Part model, mm, in its own coordinate system. A direction names the side the tool comes from. Give positions to 0.01 mm unless a question says otherwise; leave off trailing zeros. Order: outer loops, then holes, each group sorted by start corner. A loop starts at its lowest first (then second) coordinate and runs counter-clockwise, first axis right, second up. Notation, with made-up numbers: M 34,-28.5 L 84,-28.5 A21 cw 84,-14.5 Z; hole C 49,20.5 d1. An arc over 180 degrees is marked long. Answer as a JSON object with one key per item and string values.
from build123d import *

# Parameters (mm, degrees)
BOSS_EXTRUDE1_DEPTH     = 10.8
CUT_EXTRUDE1_DEPTH      = 63.509359299
CUT_EXTRUDE1_DEPTH_BACK = 63.509359299
SKETCH14_W              = 32
SKETCH14_H              = 30
CUT_EXTRUDE3_DEPTH      = 60.51688836
FILLET1_R               = 3
SKETCH16_R              = 1.6
CUT_EXTRUDE2_DEPTH      = 60.51688836
CUT_EXTRUDE4_DEPTH      = 75.590213715
BOSS_EXTRUDE3_START     = -2.5
BOSS_EXTRUDE3_OUTLINE_R = 1.65
BOSS_EXTRUDE3_DEPTH     = 2.5
BOSS_EXTRUDE4_START     = 7.1
SKETCH24_R              = 3.6
SKETCH24_R_2            = 1.6
BOSS_EXTRUDE4_DEPTH     = 7.1
CHAMFER1_SIZE           = 1


# Read off the part's stored shape, not the designer's step: Boss-Extrude3
with BuildPart() as part:
    # Sketch6 → Revolve1 (revolve)
    with BuildSketch(Plane(origin=(0, 0, 0), x_dir=(0, 0, -1), z_dir=(1, 0, 0)), mode=Mode.PRIVATE) as revolve1_sk:
        Polygon((-2, 25.4), (-2, 35.1), (-25, 35.1), (-25, 37.95), (-12, 37.95), (-12, 41.1), (-9.5, 41.1), (-9.5, 38.1), (0, 38.1), (0, 25.4), (0, 0), (-2, 0), align=None)
    revolve(revolve1_sk.sketch.rotate(Axis((0, 0, 0), (0, 0, 1)), 90), axis=Axis((0, 0, 0), (0, 0, 1)))

    # Sketch15 → Boss-Extrude1 (add)
    with BuildSketch(Plane.XY.offset(2)):
        with BuildLine():
            Line((-20, 15.904297927), (20, 15.904297927))
            ThreePointArc((20, 15.904297927), (22.121320344, 15.02561827), (23, 12.904297927))
            Line((23, 12.904297927), (23, -24.995702073))
            ThreePointArc((23, -24.995702073), (22.121320344, -27.117022417), (20, -27.995702073))
            Line((20, -27.995702073), (-20, -27.995702073))
            ThreePointArc((-20, -27.995702073), (-22.121320344, -27.117022417), (-23, -24.995702073))
            Line((-23, -24.995702073), (-23, 12.904297927))
            ThreePointArc((-23, 12.904297927), (-22.121320344, 15.02561827), (-20, 15.904297927))
        make_face()
    extrude(amount=BOSS_EXTRUDE1_DEPTH)

    # Sketch14 → Cut-Extrude1 (cut, two sides: drawn at the far end of the back side and taken through both)
    with BuildSketch(Plane.XY.offset(2).offset(-CUT_EXTRUDE1_DEPTH_BACK)):
        with Locations((-0.00164643, -5.995702073)):
            Rectangle(SKETCH14_W, SKETCH14_H)
    extrude(amount=CUT_EXTRUDE1_DEPTH + CUT_EXTRUDE1_DEPTH_BACK, mode=Mode.SUBTRACT)

    # Sketch18 → Cut-Extrude3 (cut, through all)
    with BuildSketch(Plane.XY.offset(12.8)):
        with BuildLine():
            Line((19.99835357, -24.995702073), (23.99835357, -24.995702073))
            Line((23.99835357, -24.995702073), (23.99835357, -25.995702073))
            ThreePointArc((23.99835357, -25.995702073), (23.119673914, -28.117022417), (20.99835357, -28.995702073))
            Line((20.99835357, -28.995702073), (19.99835357, -28.995702073))
            Line((19.99835357, -28.995702073), (19.99835357, -24.995702073))
        make_face()
        with BuildLine():
            Line((-20.00164643, -24.995702073), (-24.00164643, -24.995702073))
            Line((-24.00164643, -24.995702073), (-24.00164643, -25.995702073))
            ThreePointArc((-24.00164643, -25.995702073), (-23.122966774, -28.117022417), (-21.00164643, -28.995702073))
            Line((-21.00164643, -28.995702073), (-20.00164643, -28.995702073))
            Line((-20.00164643, -28.995702073), (-20.00164643, -24.995702073))
        make_face()
    extrude(amount=CUT_EXTRUDE3_DEPTH, mode=Mode.SUBTRACT)

    # Fillet1
    fillet1_edges = [part.edges().sort_by_distance(p)[0] for p in [
        (-16.00164643, 9.004297927, 6.4),
        (-16.00164643, -20.995702073, 6.4),
        (15.99835357, -20.995702073, 6.4),
        (15.99835357, 9.004297927, 6.4),
    ]]
    fillet(fillet1_edges, radius=FILLET1_R)

    # Sketch16 → Cut-Extrude2 (cut, through all)
    with BuildSketch(Plane.XY.offset(12.8)):
        with Locations((-20.00164643, 13.004297927)):
            Circle(SKETCH16_R)
        with Locations((-20.00164643, -24.995702073)):
            Circle(SKETCH16_R)
        with Locations((19.99835357, -24.995702073)):
            Circle(SKETCH16_R)
        with Locations((19.99835357, 13.004297927)):
            Circle(SKETCH16_R)
    extrude(amount=-CUT_EXTRUDE2_DEPTH, mode=Mode.SUBTRACT)

    # Sketch20 → Cut-Extrude4 (cut, through all)
    with BuildSketch(Plane(origin=(0, 15.904297927, 0), x_dir=(1, 0, 0), z_dir=(0, 1, 0))):
        Polygon((20, -12.8), (-20, -12.8), (-20, -25), (19.99835357, -25), align=None)
    extrude(amount=CUT_EXTRUDE4_DEPTH, mode=Mode.SUBTRACT)

    # Boss-Extrude3 outline → Boss-Extrude3 (add)
    # profile 1 of 2: a face of its own
    with BuildSketch(Plane.XY.offset(12).offset(BOSS_EXTRUDE3_START)):
        with BuildLine():
            Line((-26.863244514, 31.105885201), (-34.641419107, 38.884059794))
            Line((-34.641419107, 38.884059794), (-38.884059794, 34.641419107))
            Line((-38.884059794, 34.641419107), (-31.105885201, 26.863244514))
            ThreePointArc((-31.105885201, 26.863244514), (-29.062088707, 29.062088707), (-26.863244514, 31.105885201))
        make_face()
        with Locations((-34.641419107, 34.641419107)):
            Circle(BOSS_EXTRUDE3_OUTLINE_R, mode=Mode.SUBTRACT)
    # profile 2 of 2: a face of its own
    with BuildSketch(Plane.XY.offset(12).offset(BOSS_EXTRUDE3_START)):
        with BuildLine():
            Line((34.641419107, 38.884059794), (26.863244514, 31.105885201))
            ThreePointArc((26.863244514, 31.105885201), (29.062088707, 29.062088707), (31.105885201, 26.863244514))
            Line((31.105885201, 26.863244514), (38.884059794, 34.641419107))
            Line((38.884059794, 34.641419107), (34.641419107, 38.884059794))
        make_face()
        with Locations((34.641419107, 34.641419107)):
            Circle(BOSS_EXTRUDE3_OUTLINE_R, mode=Mode.SUBTRACT)
    boss_extrude3 = extrude(amount=BOSS_EXTRUDE3_DEPTH)

    # Sketch24 → Boss-Extrude4 (add)
    # profile 1 of 4: a face of its own
    with BuildSketch(Plane.XY.offset(12.8).offset(BOSS_EXTRUDE4_START)):
        with Locations(Location((-20.00164643, 13.004297927, 0), (0, 0, 213.6046846))):
            Circle(SKETCH24_R)
        with Locations((-20.00164643, 13.004297927)):
            Circle(SKETCH24_R_2, mode=Mode.SUBTRACT)
    # profile 2 of 4: a face of its own
    with BuildSketch(Plane.XY.offset(12.8).offset(BOSS_EXTRUDE4_START)):
        with Locations(Location((19.99835357, 13.004297927, 0), (0, 0, 126.336057515))):
            Circle(SKETCH24_R)
        with Locations((19.99835357, 13.004297927)):
            Circle(SKETCH24_R_2, mode=Mode.SUBTRACT)
    # profile 3 of 4: a face of its own
    with BuildSketch(Plane.XY.offset(12.8).offset(BOSS_EXTRUDE4_START)):
        with Locations(Location((-20.00164643, -24.995702073, 0), (0, 0, 198.741091164))):
            Circle(SKETCH24_R)
        with Locations((-20.00164643, -24.995702073)):
            Circle(SKETCH24_R_2, mode=Mode.SUBTRACT)
    # profile 4 of 4: a face of its own
    with BuildSketch(Plane.XY.offset(12.8).offset(BOSS_EXTRUDE4_START)):
        with Locations(Location((19.99835357, -24.995702073, 0), (0, 0, 236.442690237))):
            Circle(SKETCH24_R)
        with Locations((19.99835357, -24.995702073)):
            Circle(SKETCH24_R_2, mode=Mode.SUBTRACT)
    extrude(amount=-BOSS_EXTRUDE4_DEPTH)

    # Chamfer1
    chamfer1_edges = [part.edges().sort_by_distance(p)[0] for p in [
        (-21.60164643, 13.004297927, 19.9),
        (18.39835357, 13.004297927, 19.9),
        (-21.60164643, -24.995702073, 19.9),
        (18.39835357, -24.995702073, 19.9),
    ]]
    chamfer(chamfer1_edges, length=CHAMFER1_SIZE)

    # Mirror1: Boss-Extrude3 across plane
    add(boss_extrude3.mirror(Plane.ZX))


solid = part.part
1. Cut at B-B on x = -1. Give the cut face in (y, z), plus the area to 3 significant figures.
Worked answers:
{"outline": "M -41.09,9.5 L -38.09,9.5 L -38.09,0 L -21,0 L -21,12.8 L -28,12.8 L -28,2 L -35.09,2 L -35.09,25 L -37.94,25 L -37.94,12 L -41.09,12 Z; M 9,0 L 38.09,0 L 38.09,9.5 L 41.09,9.5 L 41.09,12 L 37.94,12 L 37.94,12.8 L 35.09,12.8 L 35.09,2 L 15.9,2 L 15.9,12.8 L 9,12.8 Z", "area": "357 mm^2"}
2. Cut at A-A on y = 0. Give the cut face in (x, z), plus the area to 3 significant figures.
Worked answers:
{"outline": "M -41.1,9.5 L -38.1,9.5 L -38.1,0 L -16,0 L -16,12.8 L -23,12.8 L -23,2 L -35.1,2 L -35.1,25 L -37.95,25 L -37.95,12 L -41.1,12 Z; M 16,0 L 38.1,0 L 38.1,9.5 L 41.1,9.5 L 41.1,12 L 37.95,12 L 37.95,25 L 35.1,25 L 35.1,2 L 23,2 L 23,12.8 L 16,12.8 Z", "area": "389 mm^2"}
3. Pin check, flat tips, straight feed: P1, Ø6, axis at x = -21.5, y = 6, coming from the +Z side; P2, Ø12, axis at x = -13, z = 19, coming from the +Y side; P3, Ø6, axis at x = 0, z = 17, coming from the -Y side. Stop position of each tip, or through.
Worked answers:
{"P1": "stops at z = 12.8", "P2": "stops at y = 16.46", "P3": "stops at y = -37.95"}
4. Which spindle directions (+Z, -Z, +X, -X, +Y, -Y) get a long thin tool onto all of the face, cutting with end or side? Do faces 1 (the cylindrical face through (15.143, -20.094, 6.49)), 2 (the flat face through (-35.05, 30.81, 10.73)), 3 (the flat face through (22.5, -27.8, 12.8)), 4 (the cylindrical face through (22.476, -26.689, 7.324)), 5 (the flat face through (34.94, 30.7, 10.73)). Say none if no direction does.
Worked answers:
{"face 1": "+Z, -Z", "face 2": "+Z, -Z, -X", "face 3": "+Z", "face 4": "none", "face 5": "+Z, -Z, +X"}
5. Probe line 1 along Y through (x, z) = (-1, 5.25); line 2 along X through (y, z) = (5, 9.25); line 3 along X through (y, z) = (10, 5.75). List the from-to ranges inside material, lowest first.
Worked answers:
{"line 1": "y = -38.09 to -35.09, -28 to -21, 9 to 15.9, 35.09 to 38.09", "line 2": "x = -37.77 to -34.74, -23 to -16, 16 to 23, 34.74 to 37.77", "line 3": "x = -36.76 to -33.65, -23 to 23, 33.65 to 36.76"}
6. Cut at C-C on y = 25. Give the cut face in (x, z), plus the area to 3 significant figures.
Worked answers:
{"outline": "M -32.62,9.5 L -28.75,9.5 L -28.75,0 L 28.75,0 L 28.75,9.5 L 32.62,9.5 L 32.62,12 L 28.55,12 L 28.55,25 L 24.64,25 L 24.64,2 L -24.64,2 L -24.64,25 L -28.55,25 L -28.55,12 L -32.62,12 Z", "area": "318 mm^2"}
